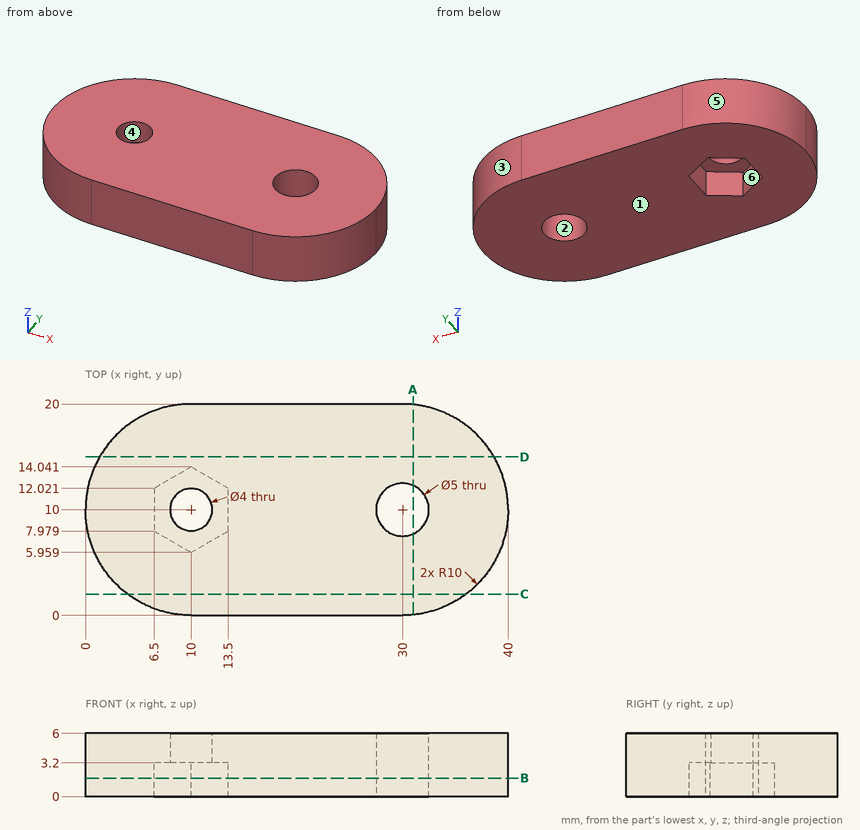
The drawing under review shows one solid part. Ordinate dimensions are in mm from its lowest x, y, z. A direction names the side the tool comes from. Round coordinates to 2 decimals unless told otherwise and drop trailing zeros. Loops run counter-clockwise (first coordinate to the right, second up) from the corner with the lowest first, then second, coordinate; pieces in that order, holes last.
Item 1: Take a section at C-C (y = 2). Write out the cut boundary in (x, z), then the cut area to 3 significant figures.
Determined:
outline: (4, 0) - (36, 0) - (36, 6) - (4, 6) - close
area: 192 mm2
Item 2: Take a section at A-A (x = 31). Write out the cut boundary in (y, z).
Determined:
outline: (0.05, 0) - (7.71, 0) - (7.71, 6) - (0.05, 6) - close; (12.29, 0) - (19.95, 0) - (19.95, 6) - (12.29, 6) - close
Item 3: Take a section at B-B (z = 1.75). Give the number of separate pieces and of enclosed holes in the cut face, then the cut area to 3 significant figures.
Determined:
separate pieces: 1
enclosed holes: 2
area: 652 mm2
Item 4: Clearance check with flat-ended pins moving along their axes: pin 1 Ø1 at (y, z) = (9, 2) entering from -X; pin 2 Ø2 at (x, y) = (9.5, 11) entering from -Z; pin 3 Ø2 at (y, z) = (3, 1.5) entering from +X. State where each tip first meets the part, or that it passes through.
Determined:
pin 1: stops at x = 0.01
pin 2: stops at z = 3.2
pin 3: stops at x = 38
Item 5: For the marked faces 5 and 6, list the 3-axis set-ups (+Z, -Z, +X, -X, +Y, -Y) from which the entire face can be reached by the end or side of a thin tool; tool diameter is ignored.
Determined:
face 5: +Z, -Z, -X, +Y
face 6: -Z
Item 6: For line 1 (Y direction, x = 10, z = 4.1); line 2 (Y direction, x = 30, z = 4.65); line 3 (X direction, y = 12.25, z = 2.55) (1 decimal), list the stretches that pass through material, from the lowest coordinate up.
Determined:
line 1: y = 0 to 8, 12 to 20
line 2: y = 0 to 7.5, 12.5 to 20
line 3: x = 0.3 to 6.9, 13.1 to 28.9, 31.1 to 39.7
Item 7: Take a section at D-D (y = 15). Write out the cut boundary in (x, z), then the cut area to 3 significant figures.
Determined:
outline: (1.34, 0) - (38.66, 0) - (38.66, 6) - (1.34, 6) - close
area: 224 mm2
Item 8: Mouldability with a two-part tool opening along X and no side actions: class the marked faces 1, 2, 3 and 4 as released by +X, released by -X, zero draft, split by the parting line, or undercut.
Determined:
face 1: zero draft
face 2: undercut
face 3: released by +X
face 4: undercut
